Autodesk Inventor part; units mm, degrees
ref_plane "YZ Plane" through (0, 0, 0) normal (1, 0, 0) x (0, 1, 0)
ref_plane "XZ Plane" through (0, 0, 0) normal (0, 1, 0) x (-1, 0, 0)
ref_plane "XY Plane" through (0, 0, 0) normal (0, 0, 1) x (1, 0, 0)
sketch "Sketch1" plane through (0, 0, 0) normal (1, 0, 0) x (0, 1, 0)
  line L0 (0, 0) -> (-36.5125, 0)
  line L1 (-36.5125, 0) -> (-36.5125, -39.6875)
  line L2 (-36.5125, -39.6875) -> (0, -39.6875)
  line L3 (0, -39.6875) -> (0, 0)
  dimension "d0" = 36.5125
  dimension "d1" = 39.6875
extrude "Extrusion1" add sketch "Sketch1" against normal blind 19.05
sketch "Sketch2" plane through (0, -36.5125, -39.6875) normal (0, 0, -1) x (-1, 0, 0)
  line L0 (0, 0) -> (0, 36.5125) construction
  line L1 (0, 0) -> (9.525, 0) construction
  line L2 (0, 0) -> (19.05, 0) construction
  line L3 (0, 0) -> (9.525, 0) construction
  line L4 (9.525, 0) -> (9.525, 1.5875) construction
  line L5 (9.525, 1.5875) -> (9.525, 8.7312) construction
  circle A0 centre (9.525, 8.7312) radius 7.1437
  dimension "d4" = 9.525
  dimension "d5" = 0
  dimension "d6" = 1.5875
  dimension "d7" = 7.1437
extrude "Extrusion2" add sketch "Sketch2" along normal blind 2.3813
sketch "Sketch3" plane through (-9.525, -27.7812, -42.0688) normal (0, 0, -1) x (-1, 0, 0)
  circle A0 centre (0, 0) radius 3.175
  point P0 (-9.525, 27.7812)
  dimension "d10" = 6.35
extrude "Extrusion3" add sketch "Sketch3" along normal blind 3.9688
sketch "Sketch4" plane through (0, -36.5125, -39.6875) normal (0, -1, 0) x (1, 0, 0)
  line L0 (0, 39.6875) -> (-6.35, 39.6875) construction
  line L1 (0, 39.6875) -> (-19.05, 39.6875)
  line L2 (-19.05, 39.6875) -> (-12.7, 39.6875) construction
  line L3 (-6.35, 39.6875) -> (-12.7, 39.6875) construction
  line L4 (-12.7, 39.6875) -> (-12.7, 36.5125)
  line L5 (-12.7, 36.5125) -> (-6.35, 36.5125)
  line L6 (-6.35, 36.5125) -> (-6.35, 39.6875)
  dimension "d13" = 6.35
  dimension "d14" = 6.35
  dimension "d15" = 3.175
extrude "Extrusion4" add sketch "Sketch4" along normal blind 6.35
properties part number "Reload_Motor"
Could you check a few things on this model? Use its own coordinates, in mm. A direction names the side the tool comes from. Give positions to 0.01 mm unless a question says otherwise; leave off trailing zeros. Order: outer loops, then holes, each group sorted by start corner. A loop starts at its lowest first (then second) coordinate and runs counter-clockwise, first axis right, second up.
1. For pin 1 (1.6 mm diameter, centred on y = -39, z = -2.5, fed in from -X); pin 2 (1.5 mm diameter, centred on x = -14.5, z = -9, fed in from -Y); pin 3 (1.6 mm diameter, centred on y = -41.5, z = -1, fed in from +X), each with a flat end and sliding along its axis, tell me the tip position at first contact or that it passes through.
Answers below:
pin 1: stops at x = -12.7
pin 2: stops at y = -36.51
pin 3: stops at x = -6.35
2. Suppose I cut it at B-B (y = -6). Write out the boundary of the cut face in (x, z), plus the area to 3 significant figures.
Answers below:
outline: (-19.05, -39.69) - (0, -39.69) - (0, 0) - (-19.05, 0) - close
area: 756 mm2
3. Which directions (+Z, -Z, +X, -X, +Y, -Y) give clear straight access to the entire face, cutting with the end or side of a thin tool? Please do faces 1 (the flat face through (-10, -40, -3.175)), 2 (the flat face through (-12.7, -40, -2)), 3 (the flat face through (-6.35, -40, -2)), 4 (the flat face through (-13, -29, -42.069)).
Answers below:
face 1: -Z, +X, -X, -Y
face 2: +Z, -Z, -X, -Y
face 3: +Z, -Z, +X, -Y
face 4: -Z
4. Suppose I cut it at A-A (x = -3.5). Write out the boundary of the cut face in (y, z).
Answers below:
outline: (-36.51, -39.69) - (-31.62, -39.69) - (-31.62, -42.07) - (-23.94, -42.07) - (-23.94, -39.69) - (0, -39.69) - (0, 0) - (-36.51, 0) - close
5. Suppose I cut it at C-C (z = -5.5). Write out the boundary of the cut face in (x, y), plus the area to 3 significant figures.
Answers below:
outline: (-19.05, -36.51) - (0, -36.51) - (0, 0) - (-19.05, 0) - close
area: 696 mm2
6. Suppose I cut it at D-D (x = -11.75). Write out the boundary of the cut face in (y, z) (1 decimal).
Answers below:
outline: (-42.9, -3.2) - (-36.5, -3.2) - (-36.5, -39.7) - (-34.6, -39.7) - (-34.6, -42.1) - (-30, -42.1) - (-30, -46) - (-25.5, -46) - (-25.5, -42.1) - (-21, -42.1) - (-21, -39.7) - (0, -39.7) - (0, 0) - (-42.9, 0) - close
7. I need wall thicknesses on L1, parallel to Y at x = -14.5, z = -37; L2, parallel to Z at x = -4.75, y = -18; L3, parallel to Z at x = -15, y = -25. Which ranges of each line are inside material? Lowest first, please.
Answers below:
L1: y = -36.51 to 0
L2: z = -39.69 to 0
L3: z = -42.07 to 0
